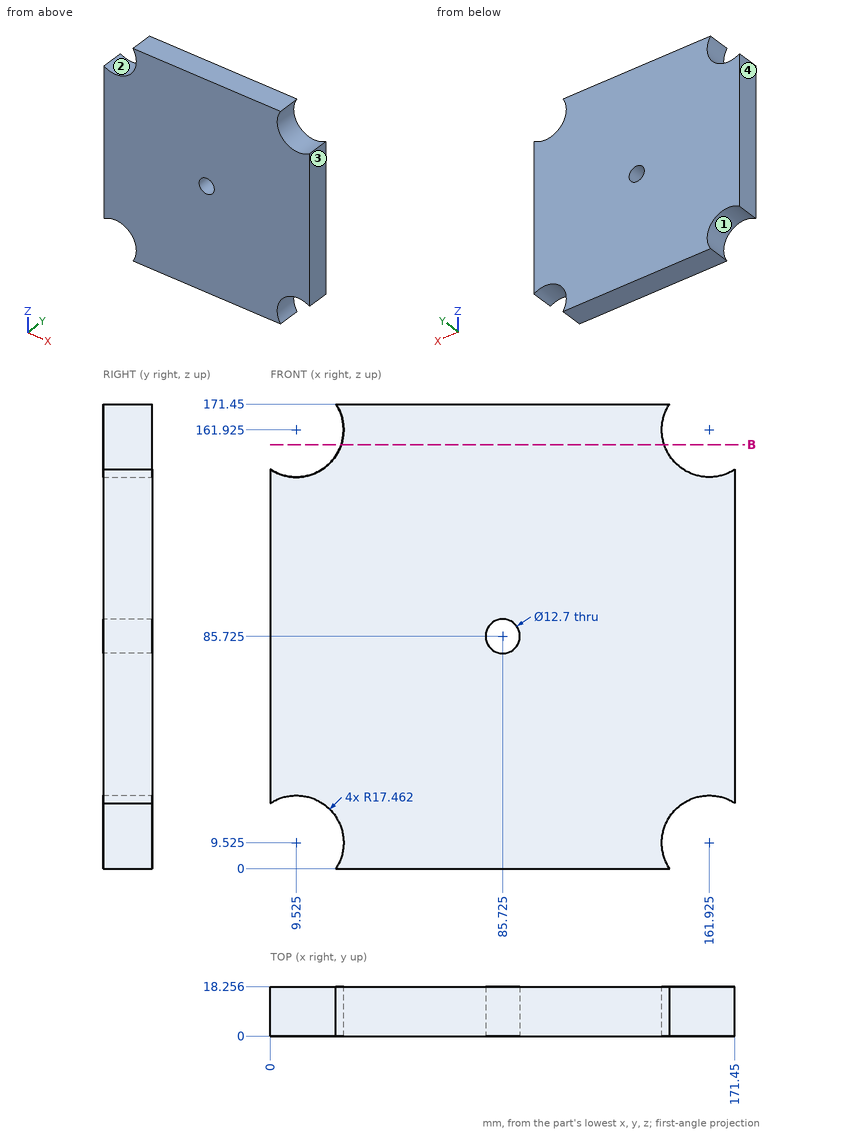
The figure shows three views and two pictorial views of one solid part (mm, origin at its lowest corner). Answer the questions. Coordinates: 2 decimals unless noted, no trailing zeros. Write each loop counter-clockwise with the first axis right and the second up, starting at its lowest first coordinate (ties: lowest second). Pieces come first, ordered by that corner, then holes.
1. Consider line 1 along Z through (x, y) = (85, 6); line 2 along Z through (x, y) = (161.5, 10). Determine where each line is inside the solid, lowest interval first.
Results list:
line 1: z = 0 to 79.42, 92.03 to 171.45
line 2: z = 26.98 to 144.47
2. The part is cut by section B-B, the plane z = 156.5. Write down the section's boundary in (x, y).
Results list:
outline: (26.12, 0) - (145.33, 0) - (145.33, 18.26) - (26.12, 18.26) - close
3. For a pull along X with two mould halves and no side action, classify the marked faces 1, 2, 3 and 4 as +X half, -X half, draft (parallel to the pull), parting line (faces both ways), or undercut.
Results list:
face 1: undercut
face 2: undercut
face 3: +X half
face 4: -X half
